from build123d import *

# Parameters (mm, degrees)
SALIENTE_EXTRUIR1_DEPTH = 372.58


with BuildPart() as part:
    # Croquis1 → Saliente-Extruir1 (new body)
    with BuildSketch(Plane(origin=(0, 0, 0), x_dir=(0, 0, -1), z_dir=(1, 0, 0))):
        with BuildLine():
            Line((38.1, 83.209074357), (0, 82.614095361))
            ThreePointArc((0, 82.614095361), (-26.940768363, 71.454863724), (-38.1, 44.514095361))
            Line((-38.1, 44.514095361), (-38.1, -31.785904639))
            ThreePointArc((-38.1, -31.785904639), (-26.940768363, -58.726673002), (0, -69.885904639))
            Line((0, -69.885904639), (38.1, -69.885904639))
            Line((38.1, -69.885904639), (38.1, 83.209074357))
        make_face()
    extrude(amount=SALIENTE_EXTRUIR1_DEPTH)


solid = part.part
Geometry check sheet. Reference: the model listing, model coordinates, mm. Give positions to 0.01 mm unless a question says otherwise; leave off trailing zeros. Order: outer loops, then holes, each group sorted by start corner. A loop starts at its lowest first (then second) coordinate and runs counter-clockwise, first axis right, second up.
1. Sectioned sample at A-A (x = 161). Record the boundary of the cut face in (y, z).
Completed:
outline: (-69.89, -38.1) - (83.21, -38.1) - (82.61, 0) arc R38.1 ccw to (44.51, 38.1) - (-31.79, 38.1) arc R38.1 ccw to (-69.89, 0) - close
2. Scan lines: line 1 (Y direction, x = 187, z = 1); line 2 (Y direction, x = 315, z = -33); line 3 (Z direction, x = 194, y = -53.5). Record each from-to range of solid material in increasing order.
Completed:
line 1: y = -69.87 to 82.6
line 2: y = -69.89 to 83.13
line 3: z = -38.1 to 31.31
3. Depth check by flat-ended pin: pin 1 (1.5 mm diameter, centred on x = 105.5, z = -15, fed in from +Y); pin 2 (12 mm diameter, centred on x = 145, z = 8.5, fed in from -Y). Enter the tip coordinate at first touch or a pass-through.
Completed:
pin 1: stops at y = 82.86
pin 2: stops at y = -69.8
